The drawing under review shows one solid part. Ordinate dimensions are in mm from its lowest x, y, z. A direction names the side the tool comes from. Round coordinates to 2 decimals unless told otherwise and drop trailing zeros. Order: outer loops, then holes, each group sorted by start corner. A loop starts at its lowest first (then second) coordinate and runs counter-clockwise, first axis right, second up. Notation, with made-up numbers: M -33.75,62.25 L 9.25,62.25 A9 cw 9.25,70.25 Z; hole C 53.25,-31.5 d2. An arc over 180 degrees is marked long. Use a Markdown table: item, result.
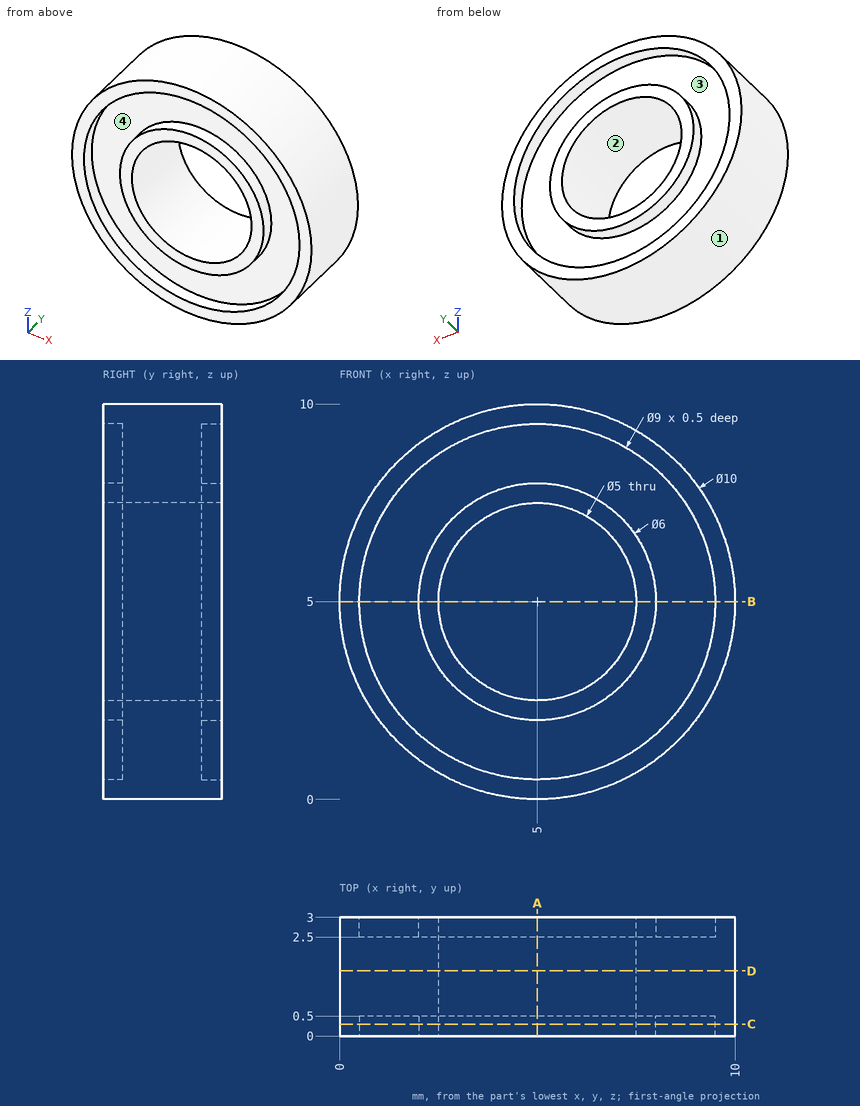
Q1. Add section B-B (z = 5). Write out the cut boundary in (x, y).
Determined:
| item | result |
|---|---|
| outline | M 0,0 L 0.5,0 L 0.5,0.5 L 2,0.5 L 2,0 L 2.5,0 L 2.5,3 L 2,3 L 2,2.5 L 0.5,2.5 L 0.5,3 L 0,3 Z; M 7.5,0 L 8,0 L 8,0.5 L 9.5,0.5 L 9.5,0 L 10,0 L 10,3 L 9.5,3 L 9.5,2.5 L 8,2.5 L 8,3 L 7.5,3 Z |
Q2. Machinability: for the marked faces 3 and 4, which of the approach directions +Z, -Z, +X, -X, +Y, -Y give a long, thin tool a straight path to every point of the face, cutting with its end or side? Answer none if there is none.
Determined:
| item | result |
|---|---|
| face 3 | +Y |
| face 4 | -Y |
Q3. Clearance check with a flat-ended pin moving along its axis: pin 1 (2.5 mm diameter, centred on x = 5, z = 5.5, fed in from +Y). State where the tip first meets the part, or that it passes through.
Determined:
| item | result |
|---|---|
| pin 1 | passes through |
Q4. Wall thickness on line 1 along Z through (x, y) = (5, 2.7); line 2 along X through (y, z) = (0.2, 6): over which ranges is each line inside the solid? List them lowest first. Write a range as [from, to].
Determined:
| item | result |
|---|---|
| line 1 | z = [0, 0.5], [2, 2.5], [7.5, 8], [9.5, 10] |
| line 2 | x = [0.1, 0.61], [2.17, 2.71], [7.29, 7.83], [9.39, 9.9] |
Q5. Add section A-A (x = 5). Write out the cut boundary in (y, z), then the cut area to 3 significant figures.
Determined:
| item | result |
|---|---|
| outline | M 0,0 L 3,0 L 3,0.5 L 2.5,0.5 L 2.5,2 L 3,2 L 3,2.5 L 0,2.5 L 0,2 L 0.5,2 L 0.5,0.5 L 0,0.5 Z; M 0,7.5 L 3,7.5 L 3,8 L 2.5,8 L 2.5,9.5 L 3,9.5 L 3,10 L 0,10 L 0,9.5 L 0.5,9.5 L 0.5,8 L 0,8 Z |
| area | 12.0 mm^2 |
Q6. Add section C-C (y = 0.3). Write out the cut boundary in (x, z).
Determined:
| item | result |
|---|---|
| outline | C 5,5 d10; C 5,5 d6; hole C 5,5 d9; hole C 5,5 d5 |
Q7. Draft analysis for pull direction X (two halves, no side actions). For the marked faces 1 and 2, state which applies: pulls with the +X half, pulls with the -X half, needs draft (parallel to the pull), parting line crosses it, or undercut.
Determined:
| item | result |
|---|---|
| face 1 | parting line crosses it |
| face 2 | undercut |
Q8. Add section D-D (y = 1.65). Write out the cut boundary in (x, z).
Determined:
| item | result |
|---|---|
| outline | C 5,5 d10; hole C 5,5 d5 |
